from build123d import *

# Parameters (mm, degrees)
SKETCH1_R           = 19.05
BOSS_EXTRUDE1_DEPTH = 4.7752
SKETCH2_R           = 9.525
BOSS_EXTRUDE2_DEPTH = 33.3248
CUT_EXTRUDE1_REACH  = 48.663
SKETCH3_R           = 2.5781
CUT_EXTRUDE2_REACH  = 48.663
SKETCH4_R           = 6
CUT_EXTRUDE3_REACH  = 48.663


with BuildPart() as part:
    # Sketch1 → Boss-Extrude1 (new body)
    with BuildSketch(Plane(origin=(0, 0, 0), x_dir=(1, 0, 0), z_dir=(0, 1, 0))):
        with Locations(Location((0, 0, 0), (0, 0, 270))):
            Circle(SKETCH1_R)
    extrude(amount=BOSS_EXTRUDE1_DEPTH)

    # Sketch2 → Boss-Extrude2 (add)
    with BuildSketch(Plane(origin=(0, 4.7752, 0), x_dir=(1, 0, 0), z_dir=(0, 1, 0))):
        with Locations(Location((0, 0, 0), (0, 0, 270))):
            Circle(SKETCH2_R)
    extrude(amount=BOSS_EXTRUDE2_DEPTH)

    # Sketch3 → Cut-Extrude1 (cut, up to next)
    with BuildSketch(Plane.XZ, mode=Mode.PRIVATE) as cut_extrude1_sk1:
        with Locations(Location((0, 14.2875, 0), (0, 0, 270))):
            Circle(SKETCH3_R)
    cut_extrude1_tool1 = extrude(cut_extrude1_sk1.sketch, amount=-CUT_EXTRUDE1_REACH, mode=Mode.PRIVATE) & part.part
    # Sketch3 → Cut-Extrude1 (cut, up to next)
    with BuildSketch(Plane.XZ, mode=Mode.PRIVATE) as cut_extrude1_sk2:
        with Locations(Location((-12.373337957, -7.14375, 0), (0, 0, 270))):
            Circle(SKETCH3_R)
    cut_extrude1_tool2 = extrude(cut_extrude1_sk2.sketch, amount=-CUT_EXTRUDE1_REACH, mode=Mode.PRIVATE) & part.part
    # Sketch3 → Cut-Extrude1 (cut, up to next)
    with BuildSketch(Plane.XZ, mode=Mode.PRIVATE) as cut_extrude1_sk3:
        with Locations(Location((12.373337957, -7.14375, 0), (0, 0, 270))):
            Circle(SKETCH3_R)
    cut_extrude1_tool3 = extrude(cut_extrude1_sk3.sketch, amount=-CUT_EXTRUDE1_REACH, mode=Mode.PRIVATE) & part.part
    add(cut_extrude1_tool1.solids().sort_by_distance((0, 0, 14.2875))[0], mode=Mode.SUBTRACT)
    add(cut_extrude1_tool2.solids().sort_by_distance((-12.373338, 0, -7.14375))[0], mode=Mode.SUBTRACT)
    add(cut_extrude1_tool3.solids().sort_by_distance((12.373338, 0, -7.14375))[0], mode=Mode.SUBTRACT)

    # Sketch4 → Cut-Extrude2 (cut, up to next)
    with BuildSketch(Plane.XZ, mode=Mode.PRIVATE) as cut_extrude2_sk1:
        with Locations(Location((0, 0, 0), (0, 0, 270))):
            Circle(SKETCH4_R)
    cut_extrude2_tool1 = extrude(cut_extrude2_sk1.sketch, amount=-CUT_EXTRUDE2_REACH, mode=Mode.PRIVATE) & part.part
    add(cut_extrude2_tool1.solids().sort_by_distance((0, 0, 0))[0], mode=Mode.SUBTRACT)

    # Sketch5 → Cut-Extrude3 (cut, up to next)
    with BuildSketch(Plane(origin=(0, 0, 0), x_dir=(-1, 0, 0), z_dir=(0, -1, 0)), mode=Mode.PRIVATE) as cut_extrude3_sk1:
        with BuildLine():
            Line((15.026391837, -11.7094), (-15.026391837, -11.7094))
            ThreePointArc((-15.026391837, -11.7094), (0, -19.05), (15.026391837, -11.7094))
        make_face()
    cut_extrude3_tool1 = extrude(cut_extrude3_sk1.sketch, amount=-CUT_EXTRUDE3_REACH, mode=Mode.PRIVATE) & part.part
    add(cut_extrude3_tool1.solids().sort_by_distance((0, 0, 14.700269))[0], mode=Mode.SUBTRACT)


solid = part.part
Input: part model. Units: mm. Frame: model coordinates. A direction names the side the tool comes from. Give positions to 0.01 mm unless a question says otherwise; leave off trailing zeros. Write each loop counter-clockwise with the first axis right and the second up, starting at its lowest first coordinate (ties: lowest second). Pieces come first, ordered by that corner, then holes. Notation, with made-up numbers: (-33.5, 67.25) -> (2.5, 67.25) arc R20 cw to (2.5, 85.25) -> close; hole circle Ø5 at (-29, -38). An arc over 180 degrees is marked (long way). Use one line per item in the form item = value. Start each with the question number.
1) Draft query along Z for faces 3 (the flat face through (-6.2, 38.1, -0.1)), 4 (the cylindrical face through (0.6, 2.35, -19.04)), 5 (the cylindrical face through (1.802, 18.783, -5.723)). Return one class per face: pulls with the +Z half, pulls with the -Z half, needs draft (parallel to the pull), parting line crosses it, or undercut.
2) Section query B-B on x = 0. Return the cut outline in (y, z) (3 decimals), then the cut area to 3 significant figures.
3) Pin query (flat end, axial travel): pin 1 (8 mm diameter, centred on x = -12.37, z = -7.14, fed in from -Y); pin 2 (12 mm diameter, centred on y = 14.5, z = -9.5, fed in from -X); pin 3 (10 mm diameter, centred on x = 14.5, z = -12, fed in from +Y); pin 4 (12 mm diameter, centred on x = 13, y = 32, fed in from +Z). Return the tip coordinate at first contact, or that it passes through.
4) Ray query, probe 1 along X at (y, z) = (19, 0) (3 decimals); probe 2 along Y at (x, z) = (-8.5, -8); probe 3 along X at (y, z) = (24.5, 2). Return the intervals inside material, ascending. Write a range as from..to.
5) Section query C-C on x = 7.5. Return the cut outline in (y, z).
6) Section query A-A on z = 0. Return the cut outline in (x, y) (3 decimals), then the cut area to 3 significant figures.
7) Set-up query: faces 1 (the flat face through (0, 4.775, -11)), 2 (the flat face through (0, 0, -7)). Return all of +Z, -Z, +X, -X, +Y, -Y with unobstructed straight access to the full face (end or side cutting, diameter ignored); none if empty.
8) Section query D-D on y = 14.5. Return the cut outline in (x, z) (3 decimals), then the cut area to 3 significant figures.
Outcome:
q1.face_3 = needs draft
q1.face_4 = parting line crosses it
q1.face_5 = undercut
q2.outline = (0, -19.05) -> (4.775, -19.05) -> (4.775, -9.525) -> (38.1, -9.525) -> (38.1, -6) -> (0, -6) -> close; (0, 6) -> (38.1, 6) -> (38.1, 9.525) -> (4.775, 9.525) -> (4.775, 11.709) -> (0, 11.709) -> close
q2.area = 325 mm^2
q3.pin_1 = 0
q3.pin_2 = -8.86
q3.pin_3 = 4.78
q3.pin_4 = 6.46
q4.probe_1 = -9.525..-6, 6..9.525
q4.probe_2 = 0..4.78
q4.probe_3 = -9.31..-5.66, 5.66..9.31
q5.outline = (0, -17.51) -> (4.78, -17.51) -> (4.78, -5.87) -> (38.1, -5.87) -> (38.1, 5.87) -> (4.78, 5.87) -> (4.78, 11.71) -> (0, 11.71) -> close
q6.outline = (-19.05, 0) -> (-6, 0) -> (-6, 38.1) -> (-9.525, 38.1) -> (-9.525, 4.775) -> (-19.05, 4.775) -> close; (6, 0) -> (19.05, 0) -> (19.05, 4.775) -> (9.525, 4.775) -> (9.525, 38.1) -> (6, 38.1) -> close
q6.area = 360 mm^2
q7.face_1 = +Y
q7.face_2 = +Z, -Z, +X, -X, -Y
q8.outline = circle Ø19.05 at (0, 0); hole circle Ø12 at (0, 0)
q8.area = 172 mm^2
